Geometry check sheet. Reference: the model listing, model coordinates, mm. Face numbers are marked on the shaded views. Coordinates: 2 decimals unless noted, no trailing zeros. Order: outer loops, then holes, each group sorted by start corner. A loop starts at its lowest first (then second) coordinate and runs counter-clockwise, first axis right, second up. Notation, with made-up numbers: (62, 3.5) - (105, 3.5) arc R13 ccw to (105, 28.5) - close; hole circle Ø2 at (-11.75, 31). An arc over 180 degrees is marked (long way). Return JSON: item names as keys, results as strings. Group by question number.
Item 1: Draft check along Y on the marked faces 1, 2 and 3. Enter one of: pulls with the +Y half, pulls with the -Y half, needs draft (parallel to the pull), parting line crosses it, or undercut.
Item 2: Section check B-B on z = 5.5. Enter the section's corners in (x, y), then the cut area to 3 significant figures.
Item 3: Gauge pin test, flat ends, axial feed: pin 1 (4 mm diameter, centred on x = -3.5, z = 18, fed in from +Y); pin 2 (1.5 mm diameter, centred on y = 3, z = 34, fed in from -X); pin 3 (1.5 mm diameter, centred on x = 1.5, z = 36, fed in from +Y). Record the tip position at first contact, or that the pin passes through.
Item 4: Section check D-D on z = 19. Enter the section's corners in (x, y), then the cut area to 3 significant figures.
Item 5: Section check A-A on x = 0. Enter the section's corners in (y, z).
Item 6: Scan lines: probe 1 along Y at (x, z) = (0, 5.25); probe 2 along Y at (x, z) = (0, 39.3); probe 3 along Z at (x, y) = (1.75, -1.5). Record each from-to range of solid material in increasing order.
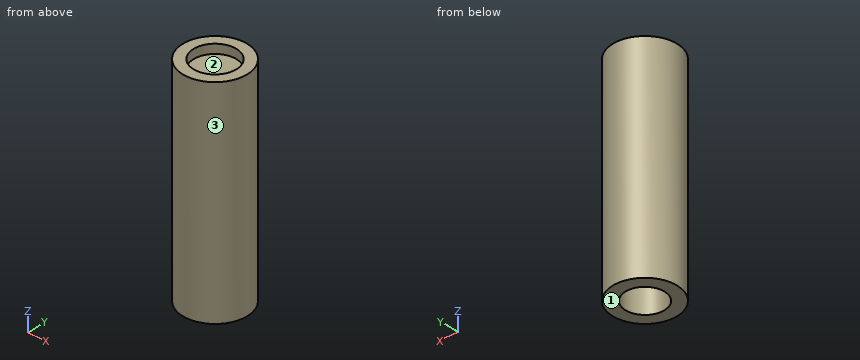
from build123d import *

# Parameters (mm, degrees)
SKETCH151_R     = 6
PAD111_DEPTH    = 40
SKETCH152_R     = 3.65
POCKET_DEPTH    = 10
SKETCH153_R     = 4
POCKET001_DEPTH = 1.7


with BuildPart() as part:
    # Sketch151 → Pad111 (new body)
    with BuildSketch(Plane.XY):
        Circle(SKETCH151_R)
    extrude(amount=PAD111_DEPTH)

    # Sketch152 (on Face2 of Pad111) → Pocket (cut)
    with BuildSketch(Plane(origin=(0, 0, 0), x_dir=(1, 0, 0), z_dir=(0, 0, -1))):
        Circle(SKETCH152_R)
    extrude(amount=-POCKET_DEPTH, mode=Mode.SUBTRACT)

    # Sketch153 (on Face3 of Pocket) → Pocket001 (cut)
    with BuildSketch(Plane.XY.offset(40)):
        Circle(SKETCH153_R)
    extrude(amount=-POCKET001_DEPTH, mode=Mode.SUBTRACT)


solid = part.part
Computed:
{
 "1": {"face 1": "needs draft", "face 2": "undercut", "face 3": "parting line crosses it"},
 "2": {"outline": "circle Ø12 at (0, 0); hole circle Ø7.3 at (0, 0)", "area": "71.2 mm²"},
 "3": {"pin 1": "stops at y = 5.81", "pin 2": "stops at x = -5.56", "pin 3": "stops at y = 5.95"},
 "4": {"outline": "circle Ø12 at (0, 0)", "area": "113 mm²"},
 "5": {"outline": "(-6, 0) - (-3.65, 0) - (-3.65, 10) - (3.65, 10) - (3.65, 0) - (6, 0) - (6, 40) - (4, 40) - (4, 38.3) - (-4, 38.3) - (-4, 40) - (-6, 40) - close"},
 "6": {"probe 1": "y = -6 to -3.65, 3.65 to 6", "probe 2": "y = -6 to -4, 4 to 6", "probe 3": "z = 10 to 38.3"}
}
